Part model, mm, in its own coordinate system. A direction names the side the tool comes from. Round coordinates to 2 decimals unless told otherwise and drop trailing zeros. Write each loop counter-clockwise with the first axis right and the second up, starting at its lowest first coordinate (ties: lowest second). Pieces come first, ordered by that corner, then holes. Notation, with made-up numbers: M 28.5,17.5 L 67.5,17.5 A16 ccw 67.5,29.5 Z; hole C -23,69 d10. An arc over 180 degrees is marked long. Use a Markdown table: item, result. Add a question column.
1) Slice it at A-A on x = 0. Write the cut outline in (y, z), plus the area to 3 significant figures.
2) Two-plate mould, pull along X, no slides. Class faces 3 (the face through (16.988, 4.424, 2.958)), 4 (the face through (4.2, 0.1, 6)), 5 (the face through (0, 19, 6)): released by +X, released by -X, zero draft, split by the parting line, or undercut.
3) Slice it at D-D on z = 10. Write the cut outline in (x, y).
4) Slice it at C-C on z = 5. Write the cut outline in (x, y).
5) Wall check: probe 1 along Y at (x, z) = (-4, 3.25); probe 2 along X at (y, z) = (18, 1); probe 3 along Y at (x, z) = (0, 4.7). Give the ranges that are in metal, low to high.
6) Which spindle directions (+Z, -Z, +X, -X, +Y, -Y) get a long thin tool onto all of the face, cutting with end or side? Do faces 1 (the face through (-13.769, 31.318, 2.958)), 2 (the face through (-1.269, 9.667, 2.958)). Say none if no direction does.
7) Drop flat-ended pins along their axis: P1, Ø4, axis at x = -3, z = 9.5, coming from the +Y side; P2, Ø2, axis at y = 13.5, z = 5, coming from the -X side; P3, Ø6, axis at y = 10, z = 5.5, coming from the +X side. Give the stop position or say it passes through.
8) Slice it at B-B on y = 25. Write the cut outline in (x, z).
```python
from build123d import *

# Parameters (mm, degrees)
CROQUIS1_R              = 9.75
SALIENTE_EXTRUIR1_DEPTH = 6
CROQUIS2_R              = 12.5
CROQUIS2_R_2            = 4
SALIENTE_EXTRUIR3_DEPTH = 7


with BuildPart() as part:
    # Croquis1 → Saliente-Extruir1 (new body)
    with BuildSketch(Plane.XY):
        with BuildLine():
            Line((-23.325317547, 15.400635095), (-10.825317547, -6.25))
            ThreePointArc((-10.825317547, -6.25), (0, -12.5), (10.825317547, -6.25))
            Line((10.825317547, -6.25), (23.325317547, 15.400635095))
            ThreePointArc((23.325317547, 15.400635095), (23.325317547, 27.900635095), (12.5, 34.150635095))
            Line((12.5, 34.150635095), (-12.5, 34.150635095))
            ThreePointArc((-12.5, 34.150635095), (-23.325317547, 27.900635095), (-23.325317547, 15.400635095))
        make_face()
        Circle(CROQUIS1_R, mode=Mode.SUBTRACT)
        with Locations((12.5, 21.650635095)):
            Circle(CROQUIS1_R, mode=Mode.SUBTRACT)
        with Locations((-12.5, 21.650635095)):
            Circle(CROQUIS1_R, mode=Mode.SUBTRACT)
    extrude(amount=SALIENTE_EXTRUIR1_DEPTH)

    # Croquis2 → Saliente-Extruir3 (add)
    with BuildSketch(Plane.XY.offset(6)):
        Circle(CROQUIS2_R)
        Circle(CROQUIS2_R_2, mode=Mode.SUBTRACT)
    extrude(amount=SALIENTE_EXTRUIR3_DEPTH)


solid = part.part
```
Entries:
| question | item | result |
|---|---|---|
| 1 | outline | M -12.5,0 L -9.75,0 L -9.75,6 L -4,6 L -4,13 L -12.5,13 Z; M 4,6 L 9.75,6 L 9.75,0 L 34.15,0 L 34.15,6 L 12.5,6 L 12.5,13 L 4,13 Z |
| 1 | area | 282 mm^2 |
| 2 | face 3 | released by +X |
| 2 | face 4 | undercut |
| 2 | face 5 | zero draft |
| 3 | outline | C 0,0 d25; hole C 0,0 d8 |
| 4 | outline | M -23.33,15.4 L -10.83,-6.25 A12.5 ccw 10.83,-6.25 L 23.33,15.4 A12.5 ccw 12.5,34.15 L -12.5,34.15 A12.5 ccw Z; hole C -12.5,21.65 d19.5; hole C 0,0 d19.5; hole C 12.5,21.65 d19.5 |
| 5 | probe 1 | y = -11.84 to -8.89, 8.89 to 16.87, 26.43 to 34.15 |
| 5 | probe 2 | x = -24.46 to -21.54, -3.46 to 3.46, 21.54 to 24.46 |
| 5 | probe 3 | y = -12.5 to -9.75, 9.75 to 34.15 |
| 6 | face 1 | +Z, -Z |
| 6 | face 2 | -Z |
| 7 | P1 | stops at y = 12.46 |
| 7 | P2 | stops at x = -22.81 |
| 7 | P3 | stops at x = 21.94 |
| 8 | outline | M -24.54,0 L -21.66,0 L -21.66,6 L -24.54,6 Z; M -3.34,0 L 3.34,0 L 3.34,6 L -3.34,6 Z; M 21.66,0 L 24.54,0 L 24.54,6 L 21.66,6 Z |
